from build123d import *

# Parameters (mm, degrees)
SKETCH1_R           = 37.5
SKETCH1_R_2         = 4
SKETCH1_R_3         = 15
BOSS_EXTRUDE1_DEPTH = 6
FILLET1_R           = 2
FILLET2_R           = 3


with BuildPart() as part:
    # Sketch1 → Boss-Extrude1 (new body)
    with BuildSketch(Plane(origin=(0, 0, 0), x_dir=(0, 0, -1), z_dir=(1, 0, 0))):
        Circle(SKETCH1_R)
        with Locations((29, 0)):
            Circle(SKETCH1_R_2, mode=Mode.SUBTRACT)
        with Locations((-14.5, -25.11473671)):
            Circle(SKETCH1_R_2, mode=Mode.SUBTRACT)
        with Locations((-14.5, 25.11473671)):
            Circle(SKETCH1_R_2, mode=Mode.SUBTRACT)
        Circle(SKETCH1_R_3, mode=Mode.SUBTRACT)
    extrude(amount=BOSS_EXTRUDE1_DEPTH)

    # Sketch2 → Revolve1 (revolve)
    with BuildSketch(Plane.XY):
        Polygon((-65, 63.5), (-70, 63.5), (-70, 54.730769231), (0, 37.5), (30.42191957, 37.5), (110, 54.476657158), (110, 63.5), (105, 63.5), (105, 57.5), (30, 41.5), (0, 41.5), (-65, 57.5), align=None)
    revolve(axis=Axis((0, 0, 0), (-1, 0, 0)))

    # Fillet1
    fillet1_edges = [part.edges().sort_by_distance(p)[0] for p in [
        (105, -57.5, 0),
        (-65, -57.5, 0),
    ]]
    fillet(fillet1_edges, radius=FILLET1_R)

    # Fillet2
    fillet2_edges = [part.edges().sort_by_distance(p)[0] for p in [
        (30, -41.5, 0),
        (0, -41.5, 0),
    ]]
    fillet(fillet2_edges, radius=FILLET2_R)


solid = part.part
Geometry: final body of the model. Coordinates: model frame, mm. A direction names the side the tool comes from. Give positions to 0.01 mm unless a question says otherwise; leave off trailing zeros. Order: outer loops, then holes, each group sorted by start corner. A loop starts at its lowest first (then second) coordinate and runs counter-clockwise, first axis right, second up. Notation, with made-up numbers: (47.5, 76.25) -> (52.5, 76.25) arc R19 ccw to (52.5, 112.25) -> close; hole circle Ø6 at (1, 88). An arc over 180 degrees is marked (long way). Answer as a JSON object with one key per item and string values.
Q1. Access query for faces 4 (the cylindrical face through (107.46, -13.77, 61.99)), 5 (the flat face through (0, -16, 1)), 6 (the conical face through (58.23, 43.9, 18.2)), 7 (the flat face through (6, 1, -16)). Directions: +Z, -Z, +X, -X, +Y, -Y. A direction counts if a zero-diameter tool reaches every point of the face in a straight line with its end or side. Return the directions, or none.
Entries:
{"face 4": "+X, -X", "face 5": "-X", "face 6": "none", "face 7": "+X"}
Q2. Draft query along Z for faces 1 (the cylindrical face through (-67.54, -13.77, 61.99)), 2 (the flat face through (110, -28, -47)), 3 (the cylindrical face through (2.958, 0.66, 14.985)). Return one class per face: released by +Z, released by -Z, zero draft, split by the parting line, or undercut.
Entries:
{"face 1": "split by the parting line", "face 2": "zero draft", "face 3": "undercut"}
Q3. Section A-A (x = 13). Output: boundary loops of the cut face in (y, z).
Entries:
{"outline": "circle Ø83 at (0, 0); hole circle Ø75 at (0, 0)"}
Q4. Material intervals for probe 1 along Z at (x, y) = (30.5, -1); probe 2 along X at (y, z) = (53.5, 25); probe 3 along Y at (x, z) = (4.3, 0), sorted ascending.
Entries:
{"probe 1": "z = -41.59 to -37.5, 37.5 to 41.59", "probe 2": "x = -70 to -65, 105 to 110", "probe 3": "y = -41.5 to -15, 15 to 41.5"}
Q5. Section B-B (y = 0). State how many separate pieces and enclosed holes the cut face has, plus the area to 3 significant figures.
Entries:
{"separate pieces": "3", "enclosed holes": "0", "area": "1,790 mm^2"}
Q6. Section C-C (x = 56.5). Output: boundary loops of the cut face in (y, z).
Entries:
{"outline": "circle Ø94.31 at (0, 0); hole circle Ø86.13 at (0, 0)"}
Q7. First-contact query: pin 1 (10 mm diameter, centred on y = 13.5, z = 15, fed in from +X); pin 2 (1 mm diameter, centred on x = 30.5, y = 16.5, fed in from +Z); pin 3 (2 mm diameter, centred on x = -30.5, y = -38, fed in from +Z); pin 4 (18 mm diameter, centred on y = 0, z = 0, fed in from +X). Flat tips, straight axial feed; report the tip coordinate or a pass-through.
Entries:
{"pin 1": "stops at x = 6", "pin 2": "stops at z = 38.44", "pin 3": "stops at z = 32.2", "pin 4": "passes through"}
